from build123d import *

# Parameters (mm, degrees)
SKETCH1_R           = 5
BOSS_EXTRUDE1_DEPTH = 15
SKETCH2_R           = 9.5
CUT_EXTRUDE1_DEPTH  = 6
SKETCH3_R           = 2
CUT_EXTRUDE2_DEPTH  = 6


with BuildPart() as part:
    # Sketch1 → Boss-Extrude1 (new body)
    with BuildSketch(Plane.XY):
        with BuildLine():
            Line((-12.5, 0), (-12.5, -10))
            Line((-12.5, -10), (-22.5, -10))
            Line((-22.5, -10), (-22.5, -15))
            Line((-22.5, -15), (22.5, -15))
            Line((22.5, -15), (22.5, -10))
            Line((22.5, -10), (12.5, -10))
            Line((12.5, -10), (12.5, 0))
            ThreePointArc((12.5, 0), (0, 12.5), (-12.5, 0))
        make_face()
        Circle(SKETCH1_R, mode=Mode.SUBTRACT)
    extrude(amount=BOSS_EXTRUDE1_DEPTH)

    # Sketch2 → Cut-Extrude1 (cut)
    with BuildSketch(Plane.XY.offset(15)):
        Circle(SKETCH2_R)
    extrude(amount=-CUT_EXTRUDE1_DEPTH, mode=Mode.SUBTRACT)

    # Sketch3 → Cut-Extrude2 (cut)
    with BuildSketch(Plane(origin=(0, -10, 0), x_dir=(1, 0, 0), z_dir=(0, 1, 0))):
        with Locations((17.5, -3.5)):
            Circle(SKETCH3_R)
        with Locations((17.5, -11.5)):
            Circle(SKETCH3_R)
        with Locations((-17.5, -11.5)):
            Circle(SKETCH3_R)
        with Locations((-17.5, -3.5)):
            Circle(SKETCH3_R)
    extrude(amount=-CUT_EXTRUDE2_DEPTH, mode=Mode.SUBTRACT)


solid = part.part
Geometry: final body of the model. Coordinates: model frame, mm. A direction names the side the tool comes from. Round coordinates to 2 decimals unless told otherwise and drop trailing zeros. Order: outer loops, then holes, each group sorted by start corner. A loop starts at its lowest first (then second) coordinate and runs counter-clockwise, first axis right, second up.
Q1. Material intervals for probe 1 along X at (y, z) = (-13.75, 3.5); probe 2 along Z at (x, y) = (-17.5, -11.85); probe 3 along Y at (x, z) = (0, 10.6), sorted ascending.
Result sheet:
probe 1: x = -22.5 to -19.5, -15.5 to 15.5, 19.5 to 22.5
probe 2: z = 0 to 1.5, 5.5 to 9.5, 13.5 to 15
probe 3: y = -15 to -9.5, 9.5 to 12.5
Q2. Section A-A, the plane z = 3.5. Output: boundary loops of the cut face in (x, y).
Result sheet:
outline: (-22.5, -15) - (-19.5, -15) - (-19.5, -10) - (-22.5, -10) - close; (-15.5, -15) - (15.5, -15) - (15.5, -10) - (12.5, -10) - (12.5, 0) arc R12.5 ccw to (-12.5, 0) - (-12.5, -10) - (-15.5, -10) - close; (19.5, -15) - (22.5, -15) - (22.5, -10) - (19.5, -10) - close; hole circle Ø10 at (0, 0)
Q3. Access query for faces 5 (the face through (18, -10, 7)), 6 (the face through (4, -4, 9)), 7 (the face through (-12.5, -5, 7)). Directions: +Z, -Z, +X, -X, +Y, -Y. A direction counts if a zero-diameter tool reaches every point of the face in a straight line with its end or side. Return the directions, or none.
Result sheet:
face 5: +Z, -Z, +X, +Y
face 6: +Z
face 7: +Z, -Z, -X, +Y
Q4. Mould query, pull axis Y, two halves, no side actions, for faces 1 (the face through (-1.08, -4.88, 4.44)), 2 (the face through (12.5, -5, 7)), 3 (the face through (-17, -10, 7)), 4 (the face through (4.38, -8.43, 12.04)). Classes: released by +Y, released by -Y, zero draft, split by the parting line, or undercut.
Result sheet:
face 1: undercut
face 2: zero draft
face 3: released by +Y
face 4: undercut
Q5. Pin query (flat end, axial travel): pin 1 (5 mm diameter, centred on x = 19.5, z = 4, fed in from +Y); pin 2 (1.5 mm diameter, centred on y = -6.5, z = 12, fed in from +X); pin 3 (2 mm diameter, centred on x = -9, y = 0, fed in from +Z); pin 4 (1.5 mm diameter, centred on y = 9.5, z = 5.5, fed in from -X). Return the tip coordinate at first contact, or that it passes through.
Result sheet:
pin 1: stops at y = -10
pin 2: stops at x = 12.5
pin 3: stops at z = 15
pin 4: stops at x = -8.93
Q6. Section D-D, the plane y = -2.5. Output: boundary loops of the cut face in (x, z), and give its area (3 significant figures).
Result sheet:
outline: (-12.5, 0) - (-4.33, 0) - (-4.33, 9) - (-9.17, 9) - (-9.17, 15) - (-12.5, 15) - close; (4.33, 0) - (12.5, 0) - (12.5, 15) - (9.17, 15) - (9.17, 9) - (4.33, 9) - close
area: 187 mm2
Q7. Section C-C, the plane z = 6.5. Output: boundary loops of the cut face in (x, y), and give its area (3 significant figures).
Result sheet:
outline: (-22.5, -15) - (22.5, -15) - (22.5, -10) - (12.5, -10) - (12.5, 0) arc R12.5 ccw to (-12.5, 0) - (-12.5, -10) - (-22.5, -10) - close; hole circle Ø10 at (0, 0)
area: 642 mm2
Q8. Section B-B, the plane x = -17.5. Output: boundary loops of the cut face in (y, z).
Result sheet:
outline: (-15, 0) - (-10, 0) - (-10, 1.5) - (-15, 1.5) - close; (-15, 5.5) - (-10, 5.5) - (-10, 9.5) - (-15, 9.5) - close; (-15, 13.5) - (-10, 13.5) - (-10, 15) - (-15, 15) - close
